from build123d import *

# Parameters (mm, degrees)
SKETCH1_R               = 2
SKETCH1_R_2             = 2.5
BOSS_EXTRUDE1_DEPTH     = 11
CUT_EXTRUDE1_REACH      = 22.585
CUT_EXTRUDE1_END_RADIUS = 2.5
SKETCH2_R               = 1.5
BOSS_EXTRUDE2_DEPTH     = 11
SKETCH4_R               = 10.9
CUT_EXTRUDE2_DEPTH      = 37.710978084


with BuildPart() as part:
    # Sketch1 → Boss-Extrude1 (new body)
    with BuildSketch(Plane(origin=(0, 0, 0), x_dir=(1, 0, 0), z_dir=(0, 1, 0))):
        with BuildLine():
            Line((-1.245136187, 9.922178988), (-40, 7.5))
            ThreePointArc((-40, 7.5), (-47.5, 0), (-40, -7.5))
            Line((-40, -7.5), (-1.245136187, -9.922178988))
            Line((-1.245136187, -9.922178988), (0, -10))
            ThreePointArc((0, -10), (10, 0), (0, 10))
            Line((0, 10), (-1.245136187, 9.922178988))
        make_face()
        with Locations(Location((-40, 0, 0), (0, 0, 270))):  # turned: the seam where the file's is
            Circle(SKETCH1_R, mode=Mode.SUBTRACT)
        with Locations(Location((0, 0, 0), (0, 0, 270))):  # turned: the seam where the file's is
            Circle(SKETCH1_R_2, mode=Mode.SUBTRACT)
    extrude(amount=BOSS_EXTRUDE1_DEPTH)

    # Cut-Extrude1: up to this cylinder (the profile starts outside it)
    cut_extrude1_end = Plane(origin=(0, 6.089956, 0), z_dir=(0, -1, 0)) * Cylinder(CUT_EXTRUDE1_END_RADIUS, 51.17, mode=Mode.PRIVATE)
    # Sketch2 → Cut-Extrude1 (cut, up to the surface)
    with BuildSketch(Plane(origin=(-0.622568093, 0, -9.961089494), x_dir=(-0.998052578, 0, 0.062378286), z_dir=(-0.062378286, 0, -0.998052578)), mode=Mode.PRIVATE) as cut_extrude1_sk1:
        with Locations(Location((0, 6.089956485, 0), (0, 0, 95.967470529))):  # turned: the seam where the file's is
            Circle(SKETCH2_R)
    cut_extrude1_tool1 = extrude(cut_extrude1_sk1.sketch, amount=-CUT_EXTRUDE1_REACH, mode=Mode.PRIVATE) - cut_extrude1_end
    add(cut_extrude1_tool1.solids().sort_by_distance((-0.622568, 6.089956, -9.961089))[0], mode=Mode.SUBTRACT)

    # Sketch3 → Boss-Extrude2 (add)
    with BuildSketch(Plane(origin=(0, 11, 0), x_dir=(1, 0, 0), z_dir=(0, 1, 0))):
        with BuildLine():
            Line((0, -17.5), (-40, -17.5))
            ThreePointArc((-40, -17.5), (-57.5, 0), (-40, 17.5))
            Line((-40, 17.5), (0, 17.5))
            ThreePointArc((0, 17.5), (17.5, 0), (0, -17.5))
        make_face()
        with BuildLine():
            Line((0, 10), (-40, 7.5))
            ThreePointArc((-40, 7.5), (-47.5, 0), (-40, -7.5))
            Line((-40, -7.5), (0, -10))
            ThreePointArc((0, -10), (10, 0), (0, 10))
        make_face(mode=Mode.SUBTRACT)
    extrude(amount=-BOSS_EXTRUDE2_DEPTH)

    # Sketch4 → Cut-Extrude2 (cut)
    with BuildSketch(Plane(origin=(0, 11, 0), x_dir=(1, 0, 0), z_dir=(0, 1, 0))):
        with Locations(Location((-40, 0, 0), (0, 0, 270))):  # turned: the seam where the file's is
            Circle(SKETCH4_R)
    extrude(amount=-CUT_EXTRUDE2_DEPTH, mode=Mode.SUBTRACT)


solid = part.part
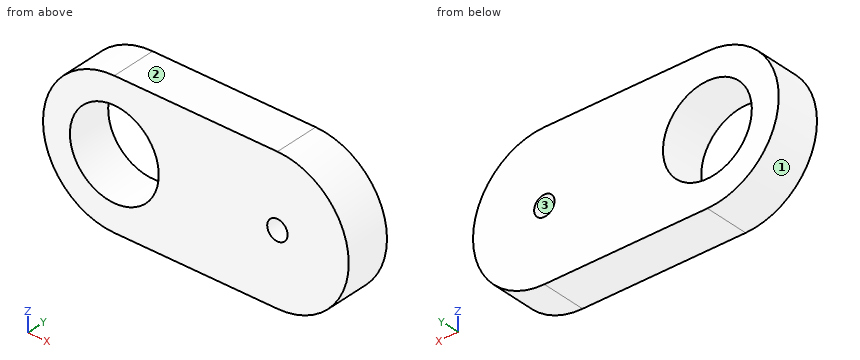
Geometry: final body of the model. Coordinates: model frame, mm. Face numbers are marked on the shaded views. Give positions to 0.01 mm unless a question says otherwise; leave off trailing zeros. Order: outer loops, then holes, each group sorted by start corner. A loop starts at its lowest first (then second) coordinate and runs counter-clockwise, first axis right, second up. Notation, with made-up numbers: (-1, 86.25) -> (35, 86.25) arc R15 ccw to (35, 107.25) -> close; hole circle Ø2 at (10, -4.75). An arc over 180 degrees is marked (long way). Answer as a JSON object with one key per item and string values.
Q1. First-contact query: pin 1 (1 mm diameter, centred on y = 4.5, z = -12.5, fed in from -X); pin 2 (1 mm diameter, centred on y = 3.5, z = -11, fed in from +X); pin 3 (4 mm diameter, centred on y = 8, z = -10, fed in from +X). Flat tips, straight axial feed; report the tip coordinate or a pass-through.
Entries:
{"pin 1": "stops at x = -52.74", "pin 2": "stops at x = 14", "pin 3": "stops at x = 15.56"}
Q2. Section B-B (x = -47). Output: boundary loops of the cut face in (y, z), plus the area to 3 significant figures.
Entries:
{"outline": "(0, -16.04) -> (11, -16.04) -> (11, -8.36) -> (0, -8.36) -> close; (0, 8.36) -> (11, 8.36) -> (11, 16.04) -> (0, 16.04) -> close", "area": "169 mm^2"}
Q3. Section D-D (z = -6.5). State how many separate pieces and enclosed holes the cut face has, plus the area to 3 significant figures.
Entries:
{"separate pieces": "2", "enclosed holes": "1", "area": "598 mm^2"}
Q4. Material intervals for probe 1 along X at (y, z) = (3, 0); probe 2 along Z at (x, y) = (-39.5, 9); probe 3 along X at (y, z) = (8.5, -0.5), sorted ascending.
Entries:
{"probe 1": "x = -57.5 to -50.9, -29.1 to -2.5, 2.5 to 17.5", "probe 2": "z = -17.5 to -10.89, 10.89 to 17.5", "probe 3": "x = -57.49 to -50.89, -29.11 to -2.45, 2.45 to 17.49"}
Q5. Draft query along X for the marked faces 1, 2 and 3. Return one class per face: released by +X, released by -X, zero draft, split by the parting line, or undercut.
Entries:
{"face 1": "released by -X", "face 2": "zero draft", "face 3": "undercut"}
Q6. Section C-C (y = 1). Output: boundary loops of the cut face in (x, z), plus the area to 3 significant figures.
Entries:
{"outline": "(-40, -17.5) -> (0, -17.5) arc R17.5 ccw to (0, 17.5) -> (-40, 17.5) arc R17.5 ccw to start; hole circle Ø21.8 at (-40, 0); hole circle Ø5 at (0, 0)", "area": "1,970 mm^2"}
Q7. Section A-A (z = 0). Output: boundary loops of the cut face in (x, y), plus the area to 3 significant figures.
Entries:
{"outline": "(-57.5, 0) -> (-50.9, 0) -> (-50.9, 11) -> (-57.5, 11) -> close; (-29.1, 0) -> (-2.5, 0) -> (-2.5, 11) -> (-29.1, 11) -> close; (2.5, 0) -> (17.5, 0) -> (17.5, 11) -> (2.5, 11) -> close", "area": "530 mm^2"}
